Design review of the part built by this model. Coordinates are the model's own, in mm. Round coordinates to 2 decimals unless told otherwise and drop trailing zeros. Order: outer loops, then holes, each group sorted by start corner. A loop starts at its lowest first (then second) coordinate and runs counter-clockwise, first axis right, second up. Notation, with made-up numbers: M -22.5,14.25 L 27.5,14.25 A34 ccw 27.5,50.25 Z; hole C -9,23 d4. An arc over 180 degrees is marked long. Use a Markdown table: item, result. Add a question column.
(1) For pin 1 (2 mm diameter, centred on y = 2, z = -1.5, fed in from -X); pin 2 (3 mm diameter, centred on x = 0, z = 0.5, fed in from -Y), all flat-tipped, find the tip position at first contact; note any pin that passes through.
(2) Take a section at C-C (x = 1.9). Write out the cut boundary in (y, z).
(3) Take a section at D-D (z = 1.6). Write out the cut boundary in (x, y).
(4) Take a section at A-A (z = 0). Write out the cut boundary in (x, y) (3 decimals), then the cut area to 3 significant figures.
(5) Take a section at B-B (x = 0). Write out the cut boundary in (y, z) (3 decimals).
(6) The part is to be moulded in two halves that separate along Z. For faces 1 (the face through (2.028, -0.754, 0.266)), 2 (the face through (0.45, 2.29, 1.43)), 3 (the face through (1, 0, -2)), say which applies: released by +Z, released by -Z, zero draft, split by the parting line, or undercut.
(7) To check wall thickness, follow probe 1 along X at (y, z) = (-1, 0) (3 decimals); probe 2 along X at (y, z) = (1.75, 0); probe 3 along Z at (x, y) = (1.3, 5.75). State the ranges of each line that lie inside material, in increasing order. Write a range as from..to.
```python
from build123d import *

# Parameters (mm, degrees)
SKETCH_1_R          = 2.78
EXTRUDE_1_DEPTH     = 6
SKETCH_2_R          = 2.045
EXTRUDE_2_DEPTH     = 1.53
CUT_EXTRUDE_1_REACH = 10.495
SKETCH_3_R          = 1.5


with BuildPart() as part:
    # 草图1 → 凸台-拉伸1 (new body)
    with BuildSketch(Plane(origin=(0, 0, 0), x_dir=(1, 0, 0), z_dir=(0, 1, 0))):
        with Locations(Location((0, 0, 0), (0, 0, 270))):
            Circle(SKETCH_1_R)
    extrude(amount=EXTRUDE_1_DEPTH)

    # 草图2 → 凸台-拉伸2 (add)
    with BuildSketch(Plane.XZ):
        with Locations(Location((0, 0, 0), (0, 0, 270))):
            Circle(SKETCH_2_R)
    extrude(amount=EXTRUDE_2_DEPTH)

    # 草图3 → 切除-拉伸1 (cut, up to next)
    with BuildSketch(Plane(origin=(0, 6, 0), x_dir=(1, 0, 0), z_dir=(0, 1, 0)), mode=Mode.PRIVATE) as cut_extrude_1_sk1:
        with Locations(Location((0, 0, 0), (0, 0, 270))):
            Circle(SKETCH_3_R)
    cut_extrude_1_tool1 = extrude(cut_extrude_1_sk1.sketch, amount=-CUT_EXTRUDE_1_REACH, mode=Mode.PRIVATE) & part.part
    add(cut_extrude_1_tool1.solids().sort_by_distance((0, 6, 0))[0], mode=Mode.SUBTRACT)


solid = part.part
```
Verdict:
| question | item | result |
|---|---|---|
| 1 | pin 1 | stops at x = -2.73 |
| 1 | pin 2 | stops at y = -1.53 |
| 2 | outline | M -1.53,-0.76 L 0,-0.76 L 0,-2.03 L 6,-2.03 L 6,2.03 L 0,2.03 L 0,0.76 L -1.53,0.76 Z |
| 3 | outline | M -2.27,0 L -1.27,0 L -1.27,-1.53 L 1.27,-1.53 L 1.27,0 L 2.27,0 L 2.27,6 L -2.27,6 Z |
| 4 | outline | M -2.78,0 L -2.045,0 L -2.045,-1.53 L -1.5,-1.53 L -1.5,6 L -2.78,6 Z; M 1.5,-1.53 L 2.045,-1.53 L 2.045,0 L 2.78,0 L 2.78,6 L 1.5,6 Z |
| 4 | area | 17.0 mm^2 |
| 5 | outline | M -1.53,-2.045 L 0,-2.045 L 0,-2.78 L 6,-2.78 L 6,-1.5 L -1.53,-1.5 Z; M -1.53,1.5 L 6,1.5 L 6,2.78 L 0,2.78 L 0,2.045 L -1.53,2.045 Z |
| 6 | face 1 | split by the parting line |
| 6 | face 2 | undercut |
| 6 | face 3 | zero draft |
| 7 | probe 1 | x = -2.045..-1.5, 1.5..2.045 |
| 7 | probe 2 | x = -2.78..-1.5, 1.5..2.78 |
| 7 | probe 3 | z = -2.46..-0.75, 0.75..2.46 |
